```python
from build123d import *

# Parameters (mm, degrees)
F1_DEPTH = 2


with BuildPart() as f1:
    # F0 (on Top) → F1 (new body)
    with BuildSketch(Plane.XY):
        with BuildLine():
            Line((26.482964, 30.72832), (-48.517036, 30.72832))
            Line((-48.517036, 30.72832), (-68.517036, 20.72832))
            Line((-68.517036, 20.72832), (-68.517036, -40.196751))
            Line((-68.517036, -40.196751), (-56.460455, -40.196751))
            Line((-56.460455, -40.196751), (-43.025967, -27.668888))
            ThreePointArc((-43.025967, -27.668888), (-22.017036, -15.27168), (-1.008104, -27.668888))
            Line((-1.008104, -27.668888), (21.482964, -48.642149))
            Line((21.482964, -48.642149), (21.482964, -65.77168))
            ThreePointArc((21.482964, -65.77168), (33.982964, -78.27168), (46.482964, -65.77168))
            Line((46.482964, -65.77168), (46.482964, -19.27168))
            ThreePointArc((46.482964, -19.27168), (31.482964, -4.27168), (46.482964, 10.72832))
            Line((46.482964, 10.72832), (46.482964, 20.72832))
            Line((46.482964, 20.72832), (26.482964, 30.72832))
        make_face()
    extrude(amount=F1_DEPTH)


solid = f1.part
```
The listing builds one solid part. Answer for the finished solid, in the listing's coordinates (mm). A direction names the side the tool comes from. Coordinates: 2 decimals unless noted, no trailing zeros. Write each loop counter-clockwise with the first axis right and the second up, starting at its lowest first coordinate (ties: lowest second). Pieces come first, ordered by that corner, then holes. Notation, with made-up numbers: M 39,56 L 63,56 A23 ccw 63,92 Z; hole C -34,74.25 d5. An arc over 180 degrees is marked long. Use a Markdown table: item, result. Add a question column.
1. For a pull along X with two mould halves and no side action, classify faces 1 (the cylindrical face through (31.487, -4.602, 0.986)), 2 (the cylindrical face through (-22.375, -15.274, 0.986)), 3 (the flat face through (10.08, -38.01, 0.99)), 4 (the cylindrical face through (33.71, -78.27, 0.99)) as +X half, -X half, draft (parallel to the pull), parting line (faces both ways), or undercut.
2. Which of the six approach directions +Z, -Z, +X, -X, +Y, -Y give full straight-line access (tool end or side, diameter ignored) to faces 5 (the flat face through (-49.837, -34.021, 0.986)), 6 (the flat face through (-12, -11, 0))?
3. Straight lines are drawn through the part: line 1 along X through (y, z) = (-50, 1.05); line 2 along X through (y, z) = (-29, 0.9); line 3 along X through (y, z) = (-27.5, 0.15). For each, find the intervals that lie inside material, in ascending order. Write a range as [from, to].
4. Section A-A (z = 0.95) is taken. Give the vertices of the cut face in (x, y).
5. Section C-C (x = -22) is taken. Give the vertices of the cut face in (y, z), plus the area to 3 significant figures.
6. Section B-B (y = -64) is taken. Give the vertices of the cut face in (x, z), plus the area to 3 significant figures.
7. Given P1, Ø1, axis at x = -60.5, z = 1, coming from the -Y side; P2, Ø0.6, axis at y = -57, z = 1, coming from the -X side, each flat-ended and moving along its own axis, determine where each tip first touches the part or whether it passes through.
Data:
| question | item | result |
|---|---|---|
| 1 | face 1 | +X half |
| 1 | face 2 | undercut |
| 1 | face 3 | undercut |
| 1 | face 4 | parting line |
| 2 | face 5 | +Z, -Z, -Y |
| 2 | face 6 | -Z, +X, -X, +Y, -Y |
| 3 | line 1 | x = [21.48, 46.48] |
| 3 | line 2 | x = [-68.52, -44.45], [0.42, 46.48] |
| 3 | line 3 | x = [-68.52, -42.93], [-1.1, 46.48] |
| 4 | outline | M -68.52,-40.2 L -56.46,-40.2 L -43.03,-27.67 A24 cw -1.01,-27.67 L 21.48,-48.64 L 21.48,-65.77 A12.5 ccw 46.48,-65.77 L 46.48,-19.27 A15 cw 46.48,10.73 L 46.48,20.73 L 26.48,30.73 L -48.52,30.73 L -68.52,20.73 Z |
| 5 | outline | M -15.27,0 L 30.73,0 L 30.73,2 L -15.27,2 Z |
| 5 | area | 92.0 mm2 |
| 6 | outline | M 21.48,0 L 46.48,0 L 46.48,2 L 21.48,2 Z |
| 6 | area | 50.0 mm2 |
| 7 | P1 | stops at y = -40.2 |
| 7 | P2 | stops at x = 21.48 |
